Design review of the part built by this model. Coordinates are the model's own, in mm. A direction names the side the tool comes from. Round coordinates to 2 decimals unless told otherwise and drop trailing zeros. Loops run counter-clockwise (first coordinate to the right, second up) from the corner with the lowest first, then second, coordinate; pieces in that order, holes last. Notation, with made-up numbers: (82, -40) -> (97, -40) arc R34 ccw to (97, -6) -> close; hole circle Ø1 at (-2.75, -6.75). An arc over 180 degrees is marked (long way). Use a Markdown table: item, result. Add a question column.
from build123d import *

# Parameters (mm, degrees)
BOSS_EXTRUDE1_DEPTH = 106.64
FILLET1_R           = 10
SHELL1_T            = -5


with BuildPart() as part:
    # Sketch1 → Boss-Extrude1 (new body)
    with BuildSketch(Plane(origin=(0, 0, 0), x_dir=(1, 0, 0), z_dir=(0, 1, 0))):
        Polygon((1.515e-14, 64.36916415), (-58.4134595853381, 64.36916415000002), (-58.4134595853381, -64.36916415000002), (1.515e-14, -64.36916415), align=None)
    extrude(amount=-BOSS_EXTRUDE1_DEPTH)

    # Sketch2 → Cut-Revolve1 (revolve, cut)
    with BuildSketch(Plane.XY):
        Polygon((-11.66115202408946, 0), (-8.083701414949179, -106.64), (-119.91640215317999, -106.64), (-119.91640215318, 0), align=None)
    revolve(axis=Axis((-119.91640215318, 0, 0), (1.3e-16, -1, 0)), mode=Mode.SUBTRACT)

    # Fillet1
    fillet1_edges = [part.edges().sort_by_distance(p)[0] for p in [
        (-14.233033878872398, -106.64, 64.36916415),
        (-14.233033878872396, -106.64, -64.36916415),
        (-16.438636834910113, 0, 64.36916415),
        (-16.43863683491015, 0, -64.36916415),
    ]]
    fillet(fillet1_edges, radius=FILLET1_R)

    # Shell1
    shell1_openings = [part.faces().sort_by_distance(p)[0] for p in [
        (-9.87242672, -53.32, 0),
        (0, -53.32, 0),
    ]]
    offset(amount=SHELL1_T, openings=shell1_openings)


solid = part.part
1. Consider section A-A on y = -93. State the section outline as (x, z) points, plus the area to 3 significant figures.
2. Mouldability with a two-part tool opening along Z and no side actions: class faces 3 (the face through (-14.64, -103.63, -61.52)), 4 (the face through (-12.95, -100.14, -57.94)), 5 (the face through (-8.142, -104.914, -0.331)), 6 (the face through (-16, -53, 64.369)) as +Z half, -Z half, draft (parallel to the pull), parting line (faces both ways), or undercut.
3. Consider section B-B on y = -70.5. State the section outline as (x, z) points.
4. To check wall thickness, follow probe 1 along Y at (x, z) = (-4.5, 48.5); probe 2 along Z at (x, y) = (-1.5, -89.5); probe 3 along Y at (x, z) = (-5, 57). State the ranges of each line that lie inside material, in increasing order. Write a range as from..to.
5. For faces 1 (the face through (-7, -5, -1)), 2 (the face through (-7, 0, -1)), list the 3-axis set-ups (+Z, -Z, +X, -X, +Y, -Y) from which the entire face can be reached by the end or side of a thin tool; tool diameter is ignored.
6. Insertion check: P1, Ø2, axis at x = -18.5, z = 29.5, coming from the +Y side. The pin has a flat end and moves straight along its axis. Give the tip position at first contact, or say it passes through.
Verdict:
| question | item | result |
|---|---|---|
| 1 | outline | (-29.03, -64.37) -> (0, -64.37) -> (0, -59.37) -> (-25.68, -59.37) arc R111.38 cw to start; (-29.03, 64.37) arc R111.38 cw to (-25.68, 59.37) -> (0, 59.37) -> (0, 64.37) -> close |
| 1 | area | 273 mm² |
| 2 | face 3 | -Z half |
| 2 | face 4 | undercut |
| 2 | face 5 | undercut |
| 2 | face 6 | +Z half |
| 3 | outline | (-29.95, -64.37) -> (0, -64.37) -> (0, -59.37) -> (-26.58, -59.37) arc R110.62 cw to start; (-29.95, 64.37) arc R110.62 cw to (-26.58, 59.37) -> (0, 59.37) -> (0, 64.37) -> close |
| 4 | probe 1 | y = -106.64..-101.64, -5..0 |
| 4 | probe 2 | z = -64.37..-59.37, 59.37..64.37 |
| 4 | probe 3 | y = -106.29..-100.89, -5.75..-0.35 |
| 5 | face 1 | +X, -X |
| 5 | face 2 | +Z, -Z, +X, -X, +Y |
| 6 | P1 | passes through |
